```python
from build123d import *

# Parameters (mm, degrees)
SKETCH1_W                  = 20
SKETCH1_H                  = 20
BOSS_EXTRUDE1_DEPTH        = 2
SKETCH2_W                  = 7
SKETCH2_H                  = 10
BOSS_EXTRUDE2_DEPTH        = 6
SKETCH3_W                  = 6.5
SKETCH3_H                  = 13
BOSS_EXTRUDE3_DEPTH        = 6
BOSS_EXTRUDE4_REACH        = 29.324
SKETCH4_W                  = 0.1
SKETCH4_H                  = 4
SKETCH5_W                  = 4
SKETCH5_H                  = 2.479052782
BOSS_EXTRUDE5_DEPTH        = 1
SKETCH6_W                  = 3
SKETCH6_H                  = 12.5
BOSS_EXTRUDE6_DEPTH        = 2
SKETCH7_W                  = 2
SKETCH7_H                  = 7
BOSS_EXTRUDE7_DEPTH        = 2
SKETCH8_W                  = 4.6
SKETCH8_H                  = 8.6
CUT_EXTRUDE1_DEPTH         = 6.3
SKETCH9_W                  = 1
SKETCH9_H                  = 1
SKETCH10_W                 = 1
SKETCH10_H                 = 1
SKETCH11_W                 = 1.55
SKETCH11_H                 = 1
SKETCH12_W                 = 1.55
SKETCH12_H                 = 1
F_3_1_3_1_DIAMETER_HOLE1_D = 3.1
RIB1_START                 = -5.8
RIB1_OUTLINE_W             = 4
RIB1_OUTLINE_H             = 4
RIB1_DEPTH                 = 11.6
FILLET1_R                  = 0.5
FILLET2_R                  = 2


# Read off the part's stored shape, not the designer's step: Rib1
with BuildPart() as part:
    # Sketch1 → Boss-Extrude1 (new body)
    with BuildSketch(Plane.XY.offset(2)):
        Rectangle(SKETCH1_W, SKETCH1_H)
    extrude(amount=-BOSS_EXTRUDE1_DEPTH)

    # Sketch2 → Boss-Extrude2 (add)
    with BuildSketch(Plane.XY.offset(2)):
        with Locations((8.5, 0)):
            Rectangle(SKETCH2_W, SKETCH2_H)
    extrude(amount=BOSS_EXTRUDE2_DEPTH)

    # Sketch3 → Boss-Extrude3 (add)
    with BuildSketch(Plane.XY.offset(2)):
        with Locations((-7.75, 1.5)):
            Rectangle(SKETCH3_W, SKETCH3_H)
    extrude(amount=BOSS_EXTRUDE3_DEPTH)

    # Boss-Extrude4: up to this plane
    boss_extrude4_end = Plane(origin=(-11, -5, 8), z_dir=(1, 0, 0))
    # Sketch4 → Boss-Extrude4 (add, up to the surface)
    with BuildSketch(Plane(origin=(-2.679775281, 11.612359551, 0), x_dir=(-0.9743911956946198, -0.22485950669875843, 0), z_dir=(-0.22485950669875843, 0.9743911956946198, 0)), mode=Mode.PRIVATE) as boss_extrude4_sk1:
        with Locations((11.567741179, 5)):
            Rectangle(SKETCH4_W, SKETCH4_H)
    boss_extrude4_tool1 = split(extrude(boss_extrude4_sk1.sketch, amount=-BOSS_EXTRUDE4_REACH, mode=Mode.PRIVATE), bisect_by=boss_extrude4_end, keep=Keep.BOTH, mode=Mode.PRIVATE)
    add(boss_extrude4_tool1.solids().sort_by_distance((-13.95128, 9.011243, 5))[0])

    # Sketch5 → Boss-Extrude5 (add)
    with BuildSketch(Plane.XY.offset(2)):
        with Locations((2, 7.760473609)):
            Rectangle(SKETCH5_W, SKETCH5_H)
    extrude(amount=BOSS_EXTRUDE5_DEPTH)

    # Sketch6 → Boss-Extrude6 (add)
    with BuildSketch(Plane(origin=(0, 0, 0), x_dir=(-1, 0, 0), z_dir=(0, 0, -1))):
        with Locations((2.5, 1.25)):
            Rectangle(SKETCH6_W, SKETCH6_H)
    extrude(amount=BOSS_EXTRUDE6_DEPTH)

    # Sketch7 → Boss-Extrude7 (add)
    with BuildSketch(Plane(origin=(0, 0, 0), x_dir=(-1, 0, 0), z_dir=(0, 0, -1))):
        with Locations((-5, 0)):
            Rectangle(SKETCH7_W, SKETCH7_H)
    extrude(amount=BOSS_EXTRUDE7_DEPTH)

    # Sketch8 → Cut-Extrude1 (cut)
    with BuildSketch(Plane(origin=(12, 0, 0), x_dir=(0, 0, -1), z_dir=(1, 0, 0))):
        with Locations((-5, 0)):
            Rectangle(SKETCH8_W, SKETCH8_H)
    extrude(amount=-CUT_EXTRUDE1_DEPTH, mode=Mode.SUBTRACT)

    # Sketch9 → Revolve1 (revolve)
    with BuildSketch(Plane(origin=(0, -1.5, 0), x_dir=(1, 0, 0), z_dir=(0, 1, 0))):
        with Locations((-5.5, 0.5)):
            Rectangle(SKETCH9_W, SKETCH9_H)
    revolve(axis=Axis((-6, -1.5, -1), (0, 0, 1)))

    # Sketch10 → Revolve2 (revolve)
    with BuildSketch(Plane(origin=(0, 5, 0), x_dir=(1, 0, 0), z_dir=(0, 1, 0))):
        with Locations((-5.5, 0.5)):
            Rectangle(SKETCH10_W, SKETCH10_H)
    revolve(axis=Axis((-6, 5, -1), (0, 0, 1)))

    # Sketch11 → Revolve3 (revolve)
    with BuildSketch(Plane.XZ.offset(-4.5), mode=Mode.PRIVATE) as revolve3_sk:
        with Locations((-4.725, 8.5)):
            Rectangle(SKETCH11_W, SKETCH11_H)
    revolve(revolve3_sk.sketch.rotate(Axis((-5.5, 4.5, 9), (0, 0, -1)), 180), axis=Axis((-5.5, 4.5, 9), (0, 0, -1)))

    # Sketch12 → Revolve4 (revolve)
    with BuildSketch(Plane.XZ.offset(2.5), mode=Mode.PRIVATE) as revolve4_sk:
        with Locations((-4.533061125, 8.5)):
            Rectangle(SKETCH12_W, SKETCH12_H)
    revolve(revolve4_sk.sketch.rotate(Axis((-5.308061125, -2.5, 9), (0, 0, -1)), 180), axis=Axis((-5.308061125, -2.5, 9), (0, 0, -1)))

    # Ø3.1 (3.1) Diameter Hole1 (through all)
    with Locations(Plane.XY.offset(2)):
        with Locations((7, -7.5), (7, 7.5)):
            Hole(F_3_1_3_1_DIAMETER_HOLE1_D / 2)

    # Rib1 outline → Rib1 (add)
    with BuildSketch(Plane(origin=(0, 1.420947218, 0), x_dir=(1, 0, 0), z_dir=(0, 1, 0)).offset(RIB1_START)):
        with Locations((-2.5, -4)):
            Rectangle(RIB1_OUTLINE_W, RIB1_OUTLINE_H)
    extrude(amount=RIB1_DEPTH)

    # Fillet1
    fillet1_edges = [part.edges().sort_by_distance(p)[0] for p in [
        (-3.95, 4.5, 9),
        (-3.758061125, -2.5, 9),
    ]]
    fillet(fillet1_edges, radius=FILLET1_R)

    # Fillet2
    fillet2_edges = [part.edges().sort_by_distance(p)[0] for p in [
        (10, 10, 1),
        (10, -10, 1),
        (-10, -10, 1),
        (-10, 10, 1),
    ]]
    fillet(fillet2_edges, radius=FILLET2_R)


solid = part.part
```
Could you check a few things on this model? Use its own coordinates, in mm. A direction names the side the tool comes from. Coordinates: 2 decimals unless noted, no trailing zeros. Write each loop counter-clockwise with the first axis right and the second up, starting at its lowest first coordinate (ties: lowest second). Pieces come first, ordered by that corner, then holes. Notation, with made-up numbers: (-7, 72) -> (35, 72) arc R26 ccw to (35, 96) -> close; hole circle Ø1 at (75.5, 3). An arc over 180 degrees is marked (long way). One line per question, with ' | ' between items. Start each with the question number.
1. If we section it at D-D (x = -10.5): Please give me the cut outline in (y, z).
2. Thinking about a two-plate mould opening in X: for faces 5 (the face through (-8, -5, 5)), 6 (the face through (-4, 1, -1)), 7 (the face through (9.4, 9.43, 0.99)), 8 (the face through (-11, 1, 5)), which applies, pulls with the +X half, pulls with the -X half, needs draft (parallel to the pull), parting line crosses it, or undercut?
3. If we section it at B-B (z = 0.5): Please give me the cut outline in (x, y).
4. If we section it at A-A (x = 7): Please give me the cut outline in (y, z).
5. Please list where these lines run through material, in increasing order: line 1 along Y through (x, z) = (7, 1.55); line 2 along X through (y, z) = (-3.25, 7.75); line 3 along Z through (x, y) = (0.75, 8).
6. Will these pins go through, and if not, where does the flat tip stop? P1, Ø5, axis at y = -7, z = 1, coming from the -X side; P2, Ø5, axis at x = -6.5, z = 6.5, coming from the +Y side; P3, Ø2, axis at x = 1, y = 5.5, coming from the -Z side.
7. For faces 1 (the face through (-6, 5, -1)), 2 (the face through (-8, 8, 5)), 3 (the face through (-3, -4.379, 4)), 4 (the face through (5.7, 0, 5)), which set-ups out of +Z, -Z, +X, -X, +Y, -Y let a thin tool reach every point of the face, with its end or its side?
8. If we section it at C-C (y = -7): Please give me the cut outline in (x, z), and give its area (3 significant figures).
Return value:
1) outline: (-5, 2) -> (8, 2) -> (8, 8) -> (-5, 8) -> close
2) face 5: needs draft | face 6: undercut | face 7: pulls with the +X half | face 8: undercut
3) outline: (-10, -8) arc R2 ccw to (-8, -10) -> (8, -10) arc R2 ccw to (10, -8) -> (10, 8) arc R2 ccw to (8, 10) -> (-8, 10) arc R2 ccw to (-10, 8) -> close; hole circle Ø3.1 at (7, -7.5); hole circle Ø3.1 at (7, 7.5)
4) outline: (-10, 0) -> (-9.05, 0) -> (-9.05, 2) -> (-10, 2) -> close; (-5.95, 0) -> (5.95, 0) -> (5.95, 2) -> (5, 2) -> (5, 8) -> (-5, 8) -> (-5, 2) -> (-5.95, 2) -> close; (9.05, 0) -> (10, 0) -> (10, 2) -> (9.05, 2) -> close; hole (-4.3, 2.7) -> (4.3, 2.7) -> (4.3, 7.3) -> (-4.3, 7.3) -> close
5) line 1: y = -10 to -9.05, -5.95 to 5.95, 9.05 to 10 | line 2: x = -11 to -4.5, 5 to 12 | line 3: z = 0 to 3
6) P1: stops at x = -11 | P2: stops at y = 8 | P3: stops at z = 0
7) face 1: -Z, -X, +Y, -Y | face 2: +Z, +Y | face 3: +Z, -Y | face 4: +X
8) outline: (-10, 0) -> (5.53, 0) -> (5.53, 2) -> (-10, 2) -> close; (8.47, 0) -> (10, 0) -> (10, 2) -> (8.47, 2) -> close | area: 34.1 mm²
